Answer from the drawing. Dimensions are ordinates in mm from the lowest x, y and z of the part. A direction names the side the tool comes from. Give positions to 0.01 mm unless a question says otherwise; leave off trailing zeros. Write each loop counter-clockwise with the first axis right and the second up, starting at its lowest first coordinate (ties: lowest second). Pieces come first, ordered by that corner, then holes.
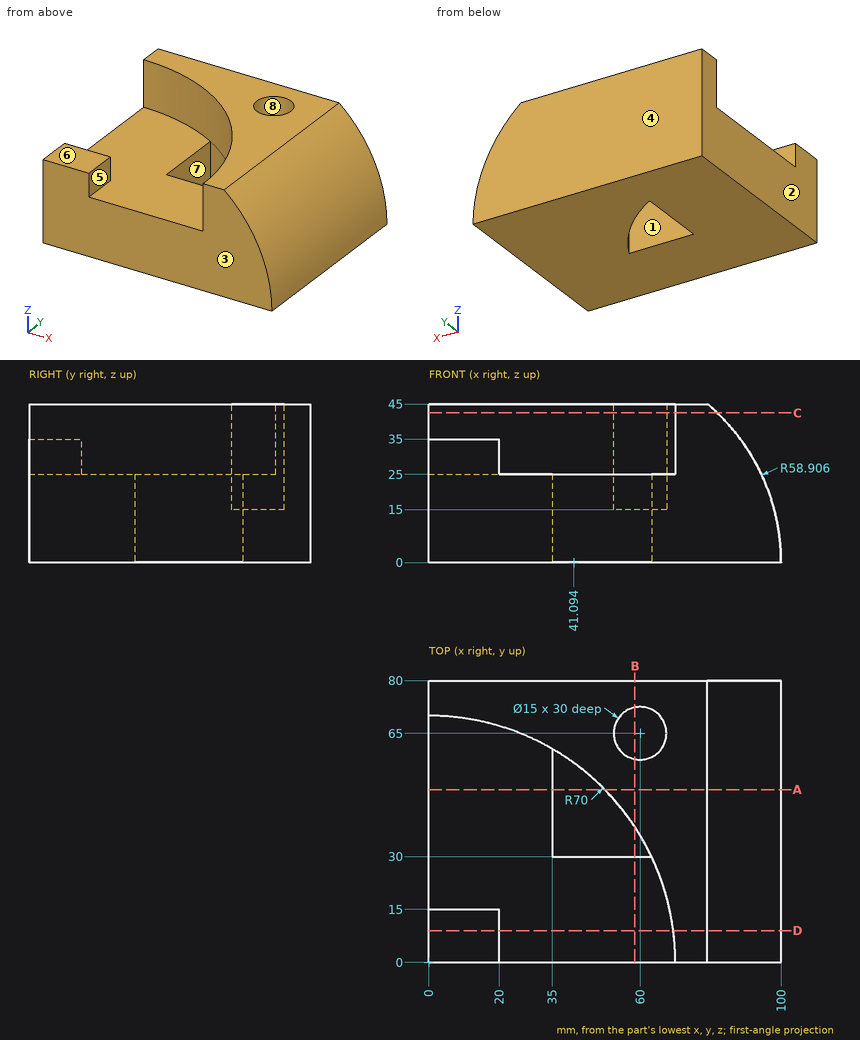
Item 1: Determine the mould class of the marked faces 1, 2 and 3 for opening direction Y: pulls with the +Y half, pulls with the -Y half, needs draft (parallel to the pull), parting line crosses it, or undercut.
Conclusion:
face 1: undercut
face 2: needs draft
face 3: pulls with the -Y half
Item 2: A cutting plane is placed at A-A, the plane y = 49. Give the vertices of the cut face in (x, z).
Conclusion:
outline: (0, 0) - (35, 0) - (35, 25) - (0, 25) - close; (49.99, 0) - (100, 0) arc R58.91 ccw to (79.11, 45) - (49.99, 45) - close
Item 3: Which of the six approach directions +Z, -Z, +X, -X, +Y, -Y give full straight-line access (tool end or side, diameter ignored) to the marked faces 4, 5, 6, 7 and 8?
Conclusion:
face 4: +Z, -Z, +X, -X, +Y
face 5: +Z, -Y
face 6: +Z, -X, -Y
face 7: +Z, -Z
face 8: +Z
Item 4: A cutting plane is placed at B-B, the plane x = 58.5. Give the vertices of the cut face in (y, z), plus the area to 3 significant figures.
Conclusion:
outline: (0, 0) - (30, 0) - (30, 25) - (0, 25) - close; (38.44, 0) - (80, 0) - (80, 45) - (72.35, 45) - (72.35, 15) - (57.65, 15) - (57.65, 45) - (38.44, 45) - close
area: 2,180 mm2
Item 5: A cutting plane is placed at C-C, the plane z = 42.5. Give the vertices of the cut face in (x, y), plus the area to 3 significant figures.
Conclusion:
outline: (0, 70) arc R70 cw to (70, 0) - (81.88, 0) - (81.88, 80) - (0, 80) - close; hole circle Ø15 at (60, 65)
area: 2,530 mm2
Item 6: A cutting plane is placed at D-D, the plane y = 9. Give the vertices of the cut face in (x, z).
Conclusion:
outline: (0, 0) - (100, 0) arc R58.91 ccw to (79.11, 45) - (69.42, 45) - (69.42, 25) - (20, 25) - (20, 35) - (0, 35) - close
Item 7: Each of these flat-tipped pins is pushed along its axis until it touches: P1, Ø1.5, axis at y = 62, z = 8, coming from the +X side; P2, Ø2, axis at y = 28.5, z = 13, coming from the +X side (1 decimal); P3, Ø12, axis at x = 12, y = 6.5, coming from the +Z side. Where does it stop, or does it pass through?
Conclusion:
P1: stops at x = 99.55
P2: stops at x = 98.8
P3: stops at z = 35
Item 8: Consider probe 1 along Y at (x, z) = (60, 22.25) (1 decimal); probe 2 along Z at (x, y) = (24, 4.5); probe 3 along Y at (x, z) = (60, 30) (1 decimal). Determine where each line is inside the solid, lowest interval first.
Conclusion:
probe 1: y = 0 to 30, 36.1 to 57.5, 72.5 to 80
probe 2: z = 0 to 25
probe 3: y = 36.1 to 57.5, 72.5 to 80
